Source: CAD feature listing. Evaluate the final solid. Frame: model axes, mm. Face numbers are marked on the shaded views. A direction names the side the tool comes from. Round coordinates to 2 decimals unless told otherwise and drop trailing zeros. Order: outer loops, then holes, each group sorted by start corner. A loop starts at its lowest first (then second) coordinate and runs counter-clockwise, first axis right, second up. Notation, with made-up numbers: (8, 11) - (60, 11) arc R30 cw to (60, 50) - close; hole circle Ø1 at (-35.75, 89). An arc over 180 degrees is marked (long way). Put each result on its own line as item: value. Start each with the question number.
1) Contact query for flat-ended pins moving along their axis: P1, Ø20.5, axis at x = 0, y = 0, coming from the +Z side; P2, Ø1.5, axis at y = -6, z = 6, coming from the +X side; P3, Ø1.6, axis at x = 16, y = -7.5, coming from the -Z side. Output: stop coordinate, or through.
2) Mould query, pull axis X, two halves, no side actions, for the marked faces 4, 5 and 6. Classes: +X half, -X half, draft (parallel to the pull), parting line (faces both ways), or undercut.
3) Section B-B on x = 0. Output: boundary loops of the cut face in (y, z), then the cut area to 3 significant figures.
4) Access query for the marked faces 1, 2 and 3. Directions: +Z, -Z, +X, -X, +Y, -Y. A direction counts if a zero-diameter tool reaches every point of the face in a straight line with its end or side. Return the directions, or none.
5) Line query: probe 1 along Y at (x, z) = (0, 5.25); probe 2 along Y at (x, z) = (0, 2.7); probe 3 along X at (y, z) = (-9, 5.5). Output: solid intervals per line, ascending. Write a range as [from, to].
6) Section A-A on y = 0. Output: boundary loops of the cut face in (x, z).
7) Section D-D on x = -4. Output: boundary loops of the cut face in (y, z).
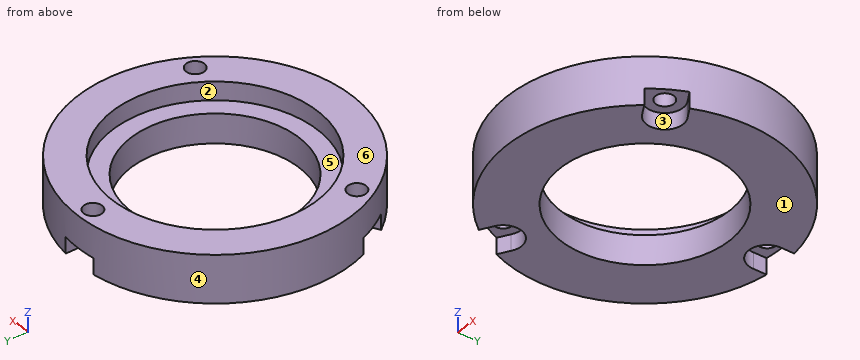
```python
from build123d import *

# Parameters (mm, degrees)
SKETCH_1_R          = 18.75
SKETCH_1_R_2        = 11.5
SKETCH_1_R_3        = 1.25
EXTRUDE_1_DEPTH     = 6.5
SKETCH_2_R          = 14
CUT_EXTRUDE_1_DEPTH = 2.5
CUT_EXTRUDE_2_DEPTH = 2.2
CUT_EXTRUDE_3_DEPTH = 2.2


with BuildPart() as part:
    # 草图1 → 凸台-拉伸1 (new body)
    with BuildSketch(Plane.XY):
        Circle(SKETCH_1_R)
        Circle(SKETCH_1_R_2, mode=Mode.SUBTRACT)
        with Locations((0, 16.75)):
            Circle(SKETCH_1_R_3, mode=Mode.SUBTRACT)
        with Locations((-14.505925513, -8.375)):
            Circle(SKETCH_1_R_3, mode=Mode.SUBTRACT)
        with Locations((14.505925513, -8.375)):
            Circle(SKETCH_1_R_3, mode=Mode.SUBTRACT)
    extrude(amount=EXTRUDE_1_DEPTH)

    # 草图2 → 切除-拉伸1 (cut)
    with BuildSketch(Plane.XY.offset(6.5)):
        Circle(SKETCH_2_R)
    extrude(amount=-CUT_EXTRUDE_1_DEPTH, mode=Mode.SUBTRACT)

    # 草图3 → 切除-拉伸2 (cut)
    with BuildSketch(Plane(origin=(0, 0, 0), x_dir=(-1, 0, 0), z_dir=(0, 0, -1))):
        with BuildLine():
            ThreePointArc((16.972613326, -7.968243025), (12.340862004, -7.125), (15.387007546, -10.714592796))
            ThreePointArc((15.387007546, -10.714592796), (16.237976321, -9.375), (16.972613326, -7.968243025))
        make_face()
        with BuildLine():
            ThreePointArc((-15.387007546, -10.714592796), (-12.340862004, -7.125), (-16.972613326, -7.968243025))
            ThreePointArc((-16.972613326, -7.968243025), (-16.237976321, -9.375), (-15.387007546, -10.714592796))
        make_face()
        with BuildLine():
            ThreePointArc((-1.58560578, 18.682835821), (0, 14.25), (1.58560578, 18.682835821))
            ThreePointArc((1.58560578, 18.682835821), (0, 18.75), (-1.58560578, 18.682835821))
        make_face()
    extrude(amount=-CUT_EXTRUDE_2_DEPTH, mode=Mode.SUBTRACT)

    # 草图4 → 切除-拉伸3 (cut)
    with BuildSketch(Plane(origin=(0, 0, 0), x_dir=(-1, 0, 0), z_dir=(0, 0, -1))):
        with BuildLine():
            Line((-14.815508707, -11.430866213), (-13.331315009, -10.581873391))
            ThreePointArc((-13.331315009, -10.581873391), (-14.344856115, -10.869805934), (-15.387007546, -10.714592796))
            ThreePointArc((-15.387007546, -10.714592796), (-15.122080143, -11.08535936), (-14.848220713, -11.449578231))
            Line((-14.848220713, -11.449578231), (-14.815508707, -11.430866213))
        make_face()
        with BuildLine():
            Line((-15.812800928, -6.24378517), (-17.28904082, -7.10668269))
            Line((-17.28904082, -7.10668269), (-17.339016827, -7.135894861))
            ThreePointArc((-17.339016827, -7.135894861), (-17.16086221, -7.554290715), (-16.972613326, -7.968243025))
            ThreePointArc((-16.972613326, -7.968243025), (-16.580385342, -6.979788038), (-15.812800928, -6.24378517))
        make_face()
        with BuildLine():
            Line((13.313677037, -10.572394724), (14.799088157, -11.419407212))
            Line((14.799088157, -11.419407212), (14.849374642, -11.448081618))
            ThreePointArc((14.849374642, -11.448081618), (15.122638772, -11.084597268), (15.387007546, -10.714592796))
            ThreePointArc((15.387007546, -10.714592796), (14.334866424, -10.869140892), (13.313677037, -10.572394724))
        make_face()
        with BuildLine():
            Line((17.339735967, -7.134147223), (17.307174882, -7.115173804))
            Line((17.307174882, -7.115173804), (15.829828681, -6.254320768))
            ThreePointArc((15.829828681, -6.254320768), (16.585956131, -6.988106842), (16.972613326, -7.968243025))
            ThreePointArc((16.972613326, -7.968243025), (17.161242887, -7.553425882), (17.339735967, -7.134147223))
        make_face()
        with BuildLine():
            Line((-2.491515254, 18.583725454), (-2.491666175, 18.546040017))
            Line((-2.491666175, 18.546040017), (-2.498513672, 16.836194159))
            ThreePointArc((-2.498513672, 16.836194159), (-2.241100016, 17.857912776), (-1.58560578, 18.682835821))
            ThreePointArc((-1.58560578, 18.682835821), (-2.039162744, 18.638785242), (-2.491515254, 18.583725454))
        make_face()
        with BuildLine():
            ThreePointArc((1.58560578, 18.682835821), (2.245518917, 17.848928929), (2.499123891, 16.816179894))
            Line((2.499123891, 16.816179894), (2.489952664, 18.526089903))
            Line((2.489952664, 18.526089903), (2.489642185, 18.58397648))
            ThreePointArc((2.489642185, 18.58397648), (2.038223439, 18.638887982), (1.58560578, 18.682835821))
        make_face()
    extrude(amount=-CUT_EXTRUDE_3_DEPTH, mode=Mode.SUBTRACT)


solid = part.part
```
Answer sheet:
1. P1: through
1. P2: x = 18
1. P3: z = 2.2
2. face 4: parting line
2. face 5: undercut
2. face 6: draft
3. outline: (-18.75, 0) - (-11.5, 0) - (-11.5, 4) - (-14, 4) - (-14, 6.5) - (-18.75, 6.5) - close; (11.5, 0) - (14.25, 0) - (14.25, 2.2) - (15.5, 2.2) - (15.5, 6.5) - (14, 6.5) - (14, 4) - (11.5, 4) - close; (18, 2.2) - (18.75, 2.2) - (18.75, 6.5) - (18, 6.5) - close
3. area: 61.1 mm^2
4. face 1: -Z, +X, -X, +Y, -Y
4. face 2: +Z
4. face 3: -Z
5. probe 1: [-18.75, -14], [14, 15.5], [18, 18.75]
5. probe 2: [-18.75, -11.5], [11.5, 15.5], [18, 18.75]
5. probe 3: [-16.45, -15.59], [-13.42, -10.72], [10.72, 13.42], [15.59, 16.45]
6. outline: (-18.75, 0) - (-11.5, 0) - (-11.5, 4) - (-14, 4) - (-14, 6.5) - (-18.75, 6.5) - close; (11.5, 0) - (18.75, 0) - (18.75, 6.5) - (14, 6.5) - (14, 4) - (11.5, 4) - close
7. outline: (-18.32, 0) - (-10.78, 0) - (-10.78, 4) - (-13.42, 4) - (-13.42, 6.5) - (-18.32, 6.5) - close; (10.78, 0) - (18.32, 0) - (18.32, 6.5) - (13.42, 6.5) - (13.42, 4) - (10.78, 4) - close
